The listing builds one solid part. Answer for the finished solid, in the listing's coordinates (mm). A direction names the side the tool comes from. Give positions to 0.01 mm unless a question says otherwise; leave off trailing zeros. Write each loop counter-clockwise with the first axis right and the second up, starting at its lowest first coordinate (ties: lowest second). Pieces come first, ordered by that corner, then holes. Notation, with made-up numbers: (62, 5) -> (82, 5) arc R22 ccw to (82, 24) -> close; hole circle Ø4 at (-38.75, 25). An arc over 180 degrees is marked (long way). Write each question's results on one line, items separated by ' | '. Start each with the question number.
Autodesk Inventor part; units mm, degrees
ref_plane "YZ Plane" through (0, 0, 0) normal (1, 0, 0) x (0, 1, 0)
ref_plane "XZ Plane" through (0, 0, 0) normal (0, 1, 0) x (-1, 0, 0)
ref_plane "XY Plane" through (0, 0, 0) normal (0, 0, 1) x (1, 0, 0)
sketch "Sketch1" plane through (0, 0, 0) normal (0, 1, 0) x (-1, 0, 0)
  line L0 (0, -5.4) -> (1.5, -5.4)
  line L1 (1.5, -5.4) -> (1.5, -8.1)
  line L2 (1.5, -8.1) -> (3.2, -8.1)
  line L3 (0, 0) -> (1.5, 0)
  line L4 (1.5, 0) -> (1.5, 2.7)
  line L5 (1.5, 2.7) -> (3.2, 2.7)
  line L6 (5, 0) -> (5, -5.4)
  line L7 (5, -5.4) -> (3.2, -8.1)
  line L8 (5, 0) -> (3.2, 2.7)
  line L9 (0, -20) -> (1.5, -20)
  line L10 (1.5, -20) -> (1.5, -17.3)
  line L11 (1.5, -17.3) -> (3.2, -17.3)
  line L12 (0, -25.4) -> (1.5, -25.4)
  line L13 (1.5, -25.4) -> (1.5, -28.1)
  line L14 (1.5, -28.1) -> (3.2, -28.1)
  line L15 (5, -20) -> (5, -25.4)
  line L16 (5, -25.4) -> (3.2, -28.1)
  line L17 (5, -20) -> (3.2, -17.3)
  line L18 (0, -5.4) -> (0, -20)
  line L19 (0, 0) -> (0, 7.3)
  line L20 (0, 7.3) -> (-5, 7.3)
  line L21 (0, -25.4) -> (0, -32.7)
  line L22 (0, -32.7) -> (-5, -32.7)
  line L23 (-5, -32.7) -> (-5, 7.3)
  dimension "d0" = 5.4
  dimension "d1" = 1.5
  dimension "d2" = 2.7
  dimension "d3" = 1.7
  dimension "d4" = 2.7
  dimension "d5" = 1.7
  dimension "d9" = 2.7
  dimension "d10" = 2.7
  dimension "d11" = 5.4
  dimension "d12" = 7.3
  dimension "d13" = 5
  dimension "d14" = 7.3
  dimension "d15" = 5
  dimension "d16" = 20
extrude "Extrusion1" add sketch "Sketch1" along normal blind 10
properties part number "slotmountingPlate_dual"
1. Section C-C (y = 1.5) is taken. Write down the section's boundary in (x, z).
2. Section B-B (z = -6) is taken. Write down the section's boundary in (x, y), then the cut area to 3 significant figures.
3. A tool of negligible diameter and unlimited length cuts with its end or side. For faces 5 (the flat face through (0, 5, -29)), 6 (the flat face through (1, 10, -12)), 7 (the flat face through (-1, 5, 0)), 8 (the flat face through (-1.5, 5, -7)), 9 (the flat face through (-2, 5, -8.1)), from which of +Z, -Z, +X, -X, +Y, -Y can it reach the whole face along a straight path? Write none if from no direction.
4. Section A-A (x = -4) is taken. Write down the section's boundary in (y, z).
5. The mould has two halves that part along X. Classify faces 1 (the flat face through (-4.113, 4.93, 1.331)), 2 (the flat face through (-2, 5, 2.7)), 3 (the flat face through (5, 5, -13)), 4 (the flat face through (-1, 5, -20)): pulls with the +X half, pulls with the -X half, needs draft (parallel to the pull), parting line crosses it, or undercut.
6. Consider probe 1 along Z at (x, y) = (-3, 8.5); probe 2 along Z at (x, y) = (-1.25, 1.75); probe 3 along X at (y, z) = (3, -29). Determine where each line is inside the solid, lowest interval first. Write a range as [from, to].
7. Each of these flat-tipped pins is pushed along its axis until it touches: pin 1 Ø0.5 at (x, y) = (-2, 7) entering from -Z; pin 2 Ø0.8 at (x, y) = (-2.5, 3.5) entering from +Z; pin 3 Ø3.5 at (y, z) = (4.5, -29.5) entering from -X. Where does it stop, or does it pass through?
8. Section D-D (z = -10) is taken. Write down the section's boundary in (x, y).
Results:
1) outline: (-5, -25.4) -> (-3.2, -28.1) -> (-1.5, -28.1) -> (-1.5, -25.4) -> (0, -25.4) -> (0, -32.7) -> (5, -32.7) -> (5, 7.3) -> (0, 7.3) -> (0, 0) -> (-1.5, 0) -> (-1.5, 2.7) -> (-3.2, 2.7) -> (-5, 0) -> (-5, -5.4) -> (-3.2, -8.1) -> (-1.5, -8.1) -> (-1.5, -5.4) -> (0, -5.4) -> (0, -20) -> (-1.5, -20) -> (-1.5, -17.3) -> (-3.2, -17.3) -> (-5, -20) -> close
2) outline: (-4.6, 0) -> (-1.5, 0) -> (-1.5, 10) -> (-4.6, 10) -> close; (0, 0) -> (5, 0) -> (5, 10) -> (0, 10) -> close | area: 81.0 mm²
3) face 5: -Z, +Y, -Y | face 6: +Z, -Z, +X, -X, +Y | face 7: +Z, +Y, -Y | face 8: +Y, -Y | face 9: -X, +Y, -Y
4) outline: (0, -26.9) -> (10, -26.9) -> (10, -18.5) -> (0, -18.5) -> close; (0, -6.9) -> (10, -6.9) -> (10, 1.5) -> (0, 1.5) -> close
5) face 1: pulls with the -X half | face 2: needs draft | face 3: pulls with the +X half | face 4: undercut
6) probe 1: z = [-28.1, -17.3], [-8.1, 2.7] | probe 2: z = [-25.4, -20], [-5.4, 0] | probe 3: x = [0, 5]
7) pin 1: stops at z = -28.1 | pin 2: stops at z = 2.7 | pin 3: stops at x = -3.43
8) outline: (0, 0) -> (5, 0) -> (5, 10) -> (0, 10) -> close
